```python
from build123d import *

# Parameters (mm, degrees)
BOSS_EXTRUDE1_DEPTH      = 26
BOSS_EXTRUDE1_DEPTH_BACK = 26
BOSS_EXTRUDE2_DEPTH      = 34
HOLE1_D                  = 18
BOSS_EXTRUDE3_DEPTH      = 22


with BuildPart() as part:
    # Sketch1 → Boss-Extrude1 (new, two sides: drawn at the far end of the back side and taken through both)
    with BuildSketch(Plane.XY.offset(-BOSS_EXTRUDE1_DEPTH_BACK)):
        with BuildLine():
            Line((-54, 34), (54, 34))
            ThreePointArc((54, 34), (88, 0), (54, -34))
            Line((54, -34), (-54, -34))
            ThreePointArc((-54, -34), (-88, 0), (-54, 34))
        make_face()
        with BuildLine():
            Line((-54, 15), (54, 15))
            ThreePointArc((54, 15), (69, 0), (54, -15))
            Line((54, -15), (-54, -15))
            ThreePointArc((-54, -15), (-69, 0), (-54, 15))
        make_face(mode=Mode.SUBTRACT)
    extrude(amount=BOSS_EXTRUDE1_DEPTH + BOSS_EXTRUDE1_DEPTH_BACK)

    # Sketch2 → Boss-Extrude2 (add)
    with BuildSketch(Plane(origin=(0, 0, -26), x_dir=(-1, 0, 0), z_dir=(0, 0, -1))):
        with BuildLine():
            Line((-29, 60), (-29, 49))
            ThreePointArc((-29, 49), (-24.606601718, 38.393398282), (-14, 34))
            Line((-14, 34), (-54, 34))
            ThreePointArc((-54, 34), (-67.647767834, 31.140623519), (-79, 23.043437244))
            Line((-79, 23.043437244), (-79, 60))
            ThreePointArc((-79, 60), (-54, 85), (-29, 60))
        make_face()
    extrude(amount=-BOSS_EXTRUDE2_DEPTH)

    # Hole1 (through all)
    with Locations(Plane(origin=(0, 0, -26), x_dir=(-1, 0, 0), z_dir=(0, 0, -1))):
        with Locations((-54, 60)):
            Hole(HOLE1_D / 2)

    # Sketch5 → Boss-Extrude3 (add)
    with BuildSketch(Plane(origin=(0, 0, -26), x_dir=(-1, 0, 0), z_dir=(0, 0, -1))):
        with BuildLine():
            Line((-14, 34), (54, 34))
            ThreePointArc((54, 34), (61.323344829, 33.201937), (68.302896095, 30.845212972))
            Line((68.302896095, 30.845212972), (-43.483164636, 82.680303656))
            ThreePointArc((-43.483164636, 82.680303656), (-32.929631184, 73.455094126), (-29, 60))
            Line((-29, 60), (-29, 49))
            ThreePointArc((-29, 49), (-24.606601718, 38.393398282), (-14, 34))
        make_face()
    extrude(amount=-BOSS_EXTRUDE3_DEPTH)


solid = part.part
```
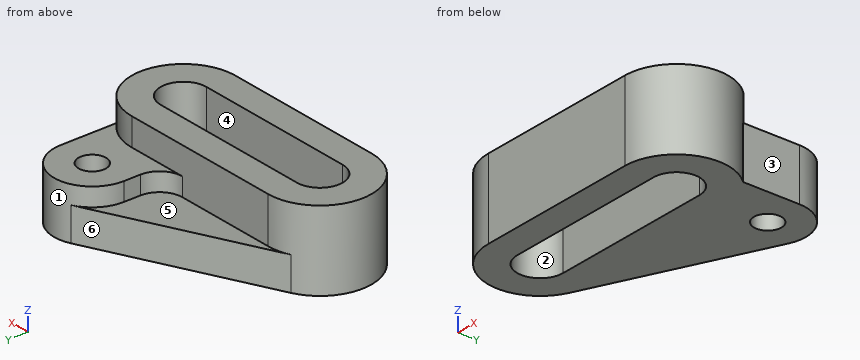
Part model, mm, in its own coordinate system. Face numbers are marked on the shaded views. A direction names the side the tool comes from. Give positions to 0.01 mm unless a question says otherwise; leave off trailing zeros. Order: outer loops, then holes, each group sorted by start corner. A loop starts at its lowest first (then second) coordinate and runs counter-clockwise, first axis right, second up. Notation, with made-up numbers: M 35,56 L 62,56 A20 ccw 62,70 Z; hole C 79,39 d5. An arc over 180 degrees is marked long. Use a Markdown table: item, result. Add a question column.
(1) Mould opens along Y. For the marked faces 4, 5 and 6 say: +Y half, -Y half, draft (parallel to the pull), parting line (faces both ways), or undercut.
(2) Saw through at A-A, the plane z = 16. Give the cut face in (x, y).
(3) Saw through at D-D, the plane x = -33. Give the cut face in (y, z), and give its area (3 significant figures).
(4) Saw through at C-C, the plane y = 0. Give the cut face in (x, z).
(5) 3-axis set-ups, long thin cutter, end or side, ignore diameter. For the marked faces 1, 2 and 3: which of +Z, -Z, +X, -X, +Y, -Y reach the whole face in a straight line?
(6) Drop flat-ended pins along their axis: P1, Ø2, axis at y = 72.5, z = -8.5, coming from the -X side; P2, Ø20.5, axis at x = 54, y = 60, coming from the +Z side; P3, Ø10, axis at y = -11.5, z = -16.5, coming from the -X side. Give the stop position or say it passes through.
(7) Saw through at B-B, the plane z = -20.5. Give the cut face in (x, y).
(8) Probe line 1 along Y through (x, z) = (54, -6.5); line 2 along Y through (x, z) = (-0.5, 20.5); line 3 along X through (y, z) = (58, 0). List the from-to ranges inside material, lowest first. Write a range as [from, to].
Answer key:
| question | item | result |
|---|---|---|
| 1 | face 4 | undercut |
| 1 | face 5 | draft |
| 1 | face 6 | +Y half |
| 2 | outline | M -54,-34 L 54,-34 A34 ccw 54,34 L -54,34 A34 ccw Z; hole M -54,-15 L 54,-15 A15 ccw 54,15 L -54,15 A15 ccw Z |
| 3 | outline | M -34,-26 L -15,-26 L -15,26 L -34,26 Z; M 15,-26 L 47.22,-26 L 47.22,-4 L 34,-4 L 34,26 L 15,26 Z |
| 3 | area | 2,270 mm^2 |
| 4 | outline | M -88,-26 L -69,-26 L -69,26 L -88,26 Z; M 69,-26 L 88,-26 L 88,26 L 69,26 Z |
| 5 | face 1 | +Z, +Y |
| 5 | face 2 | +Z, -Z |
| 5 | face 3 | +Z, -Z, +X, +Y |
| 6 | P1 | x = 19.37 |
| 6 | P2 | z = 8 |
| 6 | P3 | x = -87.37 |
| 7 | outline | M -68.3,30.85 A34 ccw -54,-34 L 54,-34 A34 ccw 79,23.04 L 79,60 A25 ccw 43.48,82.68 Z; hole M -54,-15 L 54,-15 A15 ccw 54,15 L -54,15 A15 ccw Z; hole C 54,60 d18 |
| 8 | line 1 | [-34, -15], [15, 51], [69, 85] |
| 8 | line 2 | [-34, -15], [15, 34] |
| 8 | line 3 | [29, 45.23], [62.77, 79] |
